Verification items for the finished model (mm, model axes). Face numbers are marked on the shaded views. A direction names the side the tool comes from. Coordinates: 2 decimals unless noted, no trailing zeros. Order: outer loops, then holes, each group sorted by start corner. A loop starts at its lowest first (then second) coordinate and runs counter-clockwise, first axis right, second up. Notation, with made-up numbers: M 10,55 L 24,55 A13 ccw 24,65 Z; hole C 59,56.25 d2. An arc over 180 degrees is marked long. Return JSON: item names as keys, results as strings. Group by question number.
Q1. Access from +Z, -Z, +X, -X, +Y, -Y to the whole of each face (thin tool, end or side, straight path). Record for the marked faces 1 and 2.
Q2. Mould release check, pull along X, two halves, no side actions. Record for the marked faces 3, 4 and 5: pulls with the +X half, pulls with the -X half, needs draft (parallel to the pull), parting line crosses it, or undercut.
Q3. Thickness scan on probe 1 along X at (y, z) = (9, 5). Record the ranges inside material, lowest first.
Q4. Section check C-C, the plane z = -10.75. Enter the section's corners in (x, y).
Q5. Go/stop test with a flat-tipped pin: pin 1 Ø6 at (x, y) = (5, 5.5) entering from -Z. Record where the tip stops, or that it passes through.
Q6. Section check A-A, the plane x = -6.75. Enter the section's corners in (y, z), then the cut area to 3 significant figures.
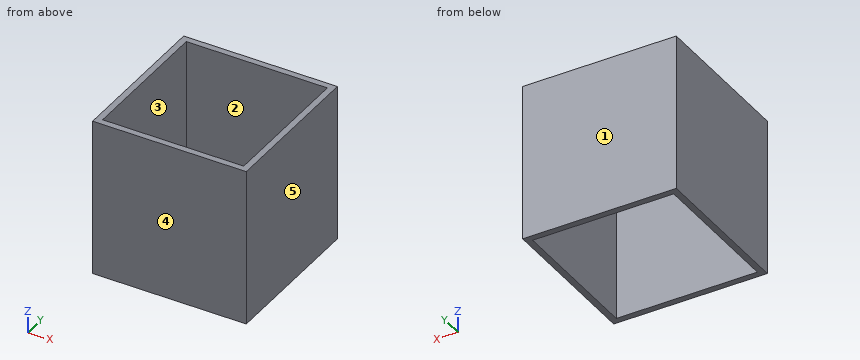
from build123d import *

# Parameters (mm, degrees)
F1_DEPTH = 12.5


with BuildPart() as f1:
    # F0 (on Top) → F1 (new body, symmetric)
    with BuildSketch(Plane.XY):
        Polygon((0.01, 12.2), (-12.2, 12.2), (-12.2, -12.2), (12.2, -12.2), (12.2, -0.1), (12.2, 12.2), align=None)
        Polygon((11.2, -11.2), (-11.2, -11.2), (-11.2, 11.2), (0, 11.2), (11.2, 11.2), (11.2, 0), align=None, mode=Mode.SUBTRACT)
    extrude(amount=F1_DEPTH, both=True)


solid = f1.part
Numbers:
{
 "1": {"face 1": "+Z, -Z, +X, -X, +Y", "face 2": "+Z, -Z"},
 "2": {"face 3": "undercut", "face 4": "needs draft", "face 5": "pulls with the +X half"},
 "3": {"probe 1": "x = -12.2 to -11.2, 11.2 to 12.2"},
 "4": {"outline": "M -12.2,-12.2 L 12.2,-12.2 L 12.2,12.2 L -12.2,12.2 Z; hole M -11.2,-11.2 L 11.2,-11.2 L 11.2,11.2 L -11.2,11.2 Z"},
 "5": {"pin 1": "passes through"},
 "6": {"outline": "M -12.2,-12.5 L -11.2,-12.5 L -11.2,12.5 L -12.2,12.5 Z; M 11.2,-12.5 L 12.2,-12.5 L 12.2,12.5 L 11.2,12.5 Z", "area": "50.0 mm2"}
}
